from build123d import *

# Parameters (mm, degrees)
ESBO_O2_R                = 2.1
RESSALTO_EXTRUS_O1_DEPTH = 14
ESBO_O3_R                = 10
RESSALTO_EXTRUS_O2_DEPTH = 5
ESBO_O4_R                = 3.50196924
CORTE_EXTRUS_O1_DEPTH    = 195
ESBO_O5_R                = 2.71004316
CORTE_EXTRUS_O2_DEPTH    = 45


with BuildPart() as part:
    # Esboço1 → Revolução1 (revolve)
    with BuildSketch(Plane.XY, mode=Mode.PRIVATE) as revolu_o1_sk:
        Polygon((9, 0), (9, -32.5), (101, -32.5), (164.919887291, -4.999614615), (222.073865158, -4.999614615), (222.073865158, 0), (164.919887291, 0), align=None)
    revolve(revolu_o1_sk.sketch.rotate(Axis((9, 0, 0), (1, 0, 0)), 270), axis=Axis((9, 0, 0), (1, 0, 0)))

    # Esboço2 → Ressalto-extrusão1 (add)
    with BuildSketch(Plane.ZY.offset(-9)):
        with Locations((0, 12.8)):
            Circle(ESBO_O2_R)
        with Locations((11.085125168, 6.4)):
            Circle(ESBO_O2_R)
        with Locations((11.085125168, -6.4)):
            Circle(ESBO_O2_R)
        with Locations((0, -12.8)):
            Circle(ESBO_O2_R)
        with Locations((-11.085125168, -6.4)):
            Circle(ESBO_O2_R)
        with Locations((-11.085125168, 6.4)):
            Circle(ESBO_O2_R)
    extrude(amount=RESSALTO_EXTRUS_O1_DEPTH)

    # Esboço3 → Ressalto-extrusão2 (add)
    with BuildSketch(Plane.ZY.offset(-9)):
        Circle(ESBO_O3_R)
    extrude(amount=RESSALTO_EXTRUS_O2_DEPTH)

    # Esboço4 → Corte-extrusão1 (cut)
    with BuildSketch(Plane(origin=(222.073865158, 0, 0), x_dir=(0, 0, -1), z_dir=(1, 0, 0))):
        Circle(ESBO_O4_R)
    extrude(amount=-CORTE_EXTRUS_O1_DEPTH, mode=Mode.SUBTRACT)

    # Esboço5 → Corte-extrusão2 (cut)
    with BuildSketch(Plane.XY):
        with Locations(Location((46.980237951, 0, 0), (0, 0, 180))):
            Circle(ESBO_O5_R)
    extrude(amount=CORTE_EXTRUS_O2_DEPTH, mode=Mode.SUBTRACT)


solid = part.part
Work out the finished part from the listing and answer in its coordinate system (mm). A direction names the side the tool comes from. Give positions to 0.01 mm unless a question says otherwise; leave off trailing zeros. Loops run counter-clockwise (first coordinate to the right, second up) from the corner with the lowest first, then second, coordinate; pieces in that order, holes last. Notation, with made-up numbers: (26, 86.5) - (33, 86.5) arc R25 cw to (33, 120.5) - close; hole circle Ø4 at (-2, 40). An arc over 180 degrees is marked (long way). Answer in a Markdown table with one row per item. Add a question column.
Q1. The part is cut by section C-C (x = 22.5). Determine the outline of the cut face in (y, z), and give its area (3 significant figures).
Q2. A tool of negligible diameter and unlimited length cuts with its end or side. For faces 4 (the cylindrical face through (2.1, 5.12, -12.75)), 5 (the flat face through (-5, 13, 0)), 6 (the cylindrical face through (125.94, 2.37, 2.58)), from which of +Z, -Z, +X, -X, +Y, -Y can it reach the whole face along a straight path? Write none if from no direction.
Q3. The part is cut by section B-B (z = 0). Determine the outline of the cut face in (x, y).
Q4. Determine the mould class of faces 1 (the cylindrical face through (6.54, -9.76, -2.17)), 2 (the flat face through (-5, 6, -11)), 3 (the cylindrical face through (2.1, -14.85, -0.46)) for opening direction Z: released by +Z, released by -Z, zero draft, split by the parting line, or undercut.
Q5. The part is cut by section A-A (y = 0). Determine the outline of the cut face in (x, z).
Q6. Each of these flat-tipped pins is pushed along its axis until it touches: P1, Ø8, axis at x = 20, z = 12, coming from the +Y side; P2, Ø1, axis at y = -25, z = -0.5, coming from the +X side; P3, Ø5, axis at x = 50.5, y = -16, coming from the +Z side. Where does it stop, or does it pass through?
Q7. Consider line 1 along Y through (x, z) = (72, 0); line 2 along Y through (x, z) = (116, 0); line 3 along Y through (x, z) = (108, 22.5). Determine where each line is inside the solid, lowest interval first.
Solution:
| question | item | result |
|---|---|---|
| 1 | outline | circle Ø65 at (0, 0) |
| 1 | area | 3,320 mm² |
| 2 | face 4 | -X |
| 2 | face 5 | +Z, -Z, -X, +Y, -Y |
| 2 | face 6 | +X |
| 3 | outline | (-5, -14.9) - (9, -14.9) - (9, -32.5) - (101, -32.5) - (164.92, -5) - (222.07, -5) - (222.07, -3.5) - (27.07, -3.5) - (27.07, 3.5) - (222.07, 3.5) - (222.07, 5) - (164.92, 5) - (101, 32.5) - (9, 32.5) - (9, 14.9) - (-5, 14.9) - (-5, 10.7) - (9, 10.7) - (9, 10) - (4, 10) - (4, -10) - (9, -10) - (9, -10.7) - (-5, -10.7) - close |
| 4 | face 1 | undercut |
| 4 | face 2 | zero draft |
| 4 | face 3 | split by the parting line |
| 5 | outline | (4, -10) - (9, -10) - (9, -32.5) - (101, -32.5) - (164.92, -5) - (222.07, -5) - (222.07, -3.5) - (27.07, -3.5) - (27.07, 3.5) - (44.27, 3.5) - (44.27, 32.5) - (9, 32.5) - (9, 10) - (4, 10) - close; (49.69, 3.5) - (222.07, 3.5) - (222.07, 5) - (164.92, 5) - (101, 32.5) - (49.69, 32.5) - close |
| 6 | P1 | stops at y = 31.5 |
| 6 | P2 | stops at x = 119.58 |
| 6 | P3 | stops at z = 29.56 |
| 7 | line 1 | y = -32.5 to -3.5, 3.5 to 32.5 |
| 7 | line 2 | y = -26.05 to -3.5, 3.5 to 26.05 |
| 7 | line 3 | y = -19.06 to 19.06 |
